```python
from build123d import *

# Parameters (mm, degrees)
SKETCH_1_W          = 18.3
SKETCH_1_H          = 42.85
SKETCH_1_R          = 1.55
EXTRUDE_1_DEPTH     = 7
SKETCH_2_W          = 5
SKETCH_2_H          = 14
EXTRUDE_4_DEPTH     = 8
SKETCH_5_W          = 5
SKETCH_5_H          = 3.15
EXTRUDE_5_DEPTH     = 35
EXTRUDE_7_DEPTH     = 35
EXTRUDE_8_DEPTH     = 5
CUT_EXTRUDE_1_REACH = 63.123
SKETCH_9_R          = 1.3
SKETCH_11_R         = 1.55
CUT_EXTRUDE_2_DEPTH = 32
SKETCH_12_W         = 6
SKETCH_12_H         = 6
CUT_EXTRUDE_3_DEPTH = 3.2
FILLET_1_R          = 5


with BuildPart() as part:
    # 草图1 → 凸台-拉伸1 (new body)
    with BuildSketch(Plane.XY):
        with Locations((9.15, -21.425)):
            Rectangle(SKETCH_1_W, SKETCH_1_H)
        with Locations((5.15, -5)):
            Circle(SKETCH_1_R, mode=Mode.SUBTRACT)
        with Locations((5.15, -37.96)):
            Circle(SKETCH_1_R, mode=Mode.SUBTRACT)
        with Locations(Location((13.15, -37.96, 0), (0, 0, 180))):
            Circle(SKETCH_1_R, mode=Mode.SUBTRACT)
        with Locations(Location((13.15, -5, 0), (0, 0, 180))):
            Circle(SKETCH_1_R, mode=Mode.SUBTRACT)
    extrude(amount=EXTRUDE_1_DEPTH)

    # 草图2 → 凸台-拉伸4 (add)
    with BuildSketch(Plane.XY.offset(7)):
        with Locations((15.8, -21.425)):
            Rectangle(SKETCH_2_W, SKETCH_2_H)
    extrude(amount=EXTRUDE_4_DEPTH)

    # 草图5 → 凸台-拉伸5 (add)
    with BuildSketch(Plane.XY.offset(7)):
        with Locations((15.8, -32.45)):
            Rectangle(SKETCH_5_W, SKETCH_5_H)
        with Locations((15.8, -10.4)):
            Rectangle(SKETCH_5_W, SKETCH_5_H)
    extrude(amount=EXTRUDE_5_DEPTH)

    # 草图7 → 凸台-拉伸7 (add)
    with BuildSketch(Plane.XY.offset(7)):
        Polygon((0, 0), (12.7, 0), (18.3, 0), (18.3, -8.825), (11.66, -8.825), (11.66, -34.025), (18.3, -34.025), (18.3, -42.85), (12.7, -42.85), (0, -42.85), align=None)
    extrude(amount=EXTRUDE_7_DEPTH)

    # 草图8 → 凸台-拉伸8 (add)
    with BuildSketch(Plane.XY.offset(7)):
        Polygon((13.3, -30.875), (13.3, -34.025), (11.66, -34.025), (11.66, -8.825), (13.3, -8.825), (13.3, -11.975), (18.3, -11.975), (18.3, -14.425), (13.3, -14.425), (13.3, -28.425), (18.3, -28.425), (18.3, -30.875), align=None)
    extrude(amount=EXTRUDE_8_DEPTH)

    # 草图9 → 切除-拉伸1 (cut, up to next)
    with BuildSketch(Plane(origin=(11.66, 0, 0), x_dir=(0, 0, -1), z_dir=(1, 0, 0)), mode=Mode.PRIVATE) as cut_extrude_1_sk1:
        with Locations(Location((-16.37, -13.195, 0), (0, 0, 90))):
            Circle(SKETCH_9_R)
    cut_extrude_1_tool1 = extrude(cut_extrude_1_sk1.sketch, amount=-CUT_EXTRUDE_1_REACH, mode=Mode.PRIVATE) & part.part
    # 草图9 → 切除-拉伸1 (cut, up to next)
    with BuildSketch(Plane(origin=(11.66, 0, 0), x_dir=(0, 0, -1), z_dir=(1, 0, 0)), mode=Mode.PRIVATE) as cut_extrude_1_sk2:
        with Locations((-16.37, -29.655)):
            Circle(SKETCH_9_R)
    cut_extrude_1_tool2 = extrude(cut_extrude_1_sk2.sketch, amount=-CUT_EXTRUDE_1_REACH, mode=Mode.PRIVATE) & part.part
    # 草图9 → 切除-拉伸1 (cut, up to next)
    with BuildSketch(Plane(origin=(11.66, 0, 0), x_dir=(0, 0, -1), z_dir=(1, 0, 0)), mode=Mode.PRIVATE) as cut_extrude_1_sk3:
        with Locations(Location((-32.63, -13.195, 0), (0, 0, 90))):
            Circle(SKETCH_9_R)
    cut_extrude_1_tool3 = extrude(cut_extrude_1_sk3.sketch, amount=-CUT_EXTRUDE_1_REACH, mode=Mode.PRIVATE) & part.part
    # 草图9 → 切除-拉伸1 (cut, up to next)
    with BuildSketch(Plane(origin=(11.66, 0, 0), x_dir=(0, 0, -1), z_dir=(1, 0, 0)), mode=Mode.PRIVATE) as cut_extrude_1_sk4:
        with Locations((-32.63, -29.655)):
            Circle(SKETCH_9_R)
    cut_extrude_1_tool4 = extrude(cut_extrude_1_sk4.sketch, amount=-CUT_EXTRUDE_1_REACH, mode=Mode.PRIVATE) & part.part
    add(cut_extrude_1_tool1.solids().sort_by_distance((11.66, -13.195, 16.37))[0], mode=Mode.SUBTRACT)
    add(cut_extrude_1_tool2.solids().sort_by_distance((11.66, -29.655, 16.37))[0], mode=Mode.SUBTRACT)
    add(cut_extrude_1_tool3.solids().sort_by_distance((11.66, -13.195, 32.63))[0], mode=Mode.SUBTRACT)
    add(cut_extrude_1_tool4.solids().sort_by_distance((11.66, -29.655, 32.63))[0], mode=Mode.SUBTRACT)

    # 草图11 → 切除-拉伸2 (cut)
    with BuildSketch(Plane(origin=(0, 0, 0), x_dir=(-1, 0, 0), z_dir=(0, 0, -1))):
        with Locations((-13.15, -5)):
            Circle(SKETCH_11_R)
        with Locations((-5.15, -5)):
            Circle(SKETCH_11_R)
        with Locations((-5.15, -37.96)):
            Circle(SKETCH_11_R)
        with Locations((-13.15, -37.96)):
            Circle(SKETCH_11_R)
    extrude(amount=-CUT_EXTRUDE_2_DEPTH, mode=Mode.SUBTRACT)

    # 草图12 → 切除-拉伸3 (cut)
    with BuildSketch(Plane.XY.offset(25)):
        with Locations((13.15, -5)):
            Rectangle(SKETCH_12_W, SKETCH_12_H)
        with Locations((5.15, -5)):
            Rectangle(SKETCH_12_W, SKETCH_12_H)
        with Locations((13.15, -37.96)):
            Rectangle(SKETCH_12_W, SKETCH_12_H)
        with Locations((5.15, -37.96)):
            Rectangle(SKETCH_12_W, SKETCH_12_H)
    extrude(amount=-CUT_EXTRUDE_3_DEPTH, mode=Mode.SUBTRACT)

    # 圆角1
    fillet_1_edges = [part.edges().sort_by_distance(p)[0] for p in [
        (9.15, -42.85, 42),
        (18.3, 0, 21),
        (18.3, -42.85, 21),
        (9.15, 0, 42),
    ]]
    fillet(fillet_1_edges, radius=FILLET_1_R)


solid = part.part
```
The model under review builds one solid part; all positions refer to its coordinate system, in mm. A direction names the side the tool comes from. Round coordinates to 2 decimals unless told otherwise and drop trailing zeros. Order: outer loops, then holes, each group sorted by start corner. A loop starts at its lowest first (then second) coordinate and runs counter-clockwise, first axis right, second up.
Item 1: Add section A-A, the plane z = 20.5. State the section outline as (x, y) points (3 decimals), and give its area (3 significant figures).
Working result:
outline: (0, -42.85) - (13.3, -42.85) arc R5 ccw to (18.3, -37.85) - (18.3, -30.875) - (13.3, -30.875) - (13.3, -34.025) - (11.66, -34.025) - (11.66, -8.825) - (13.3, -8.825) - (13.3, -11.975) - (18.3, -11.975) - (18.3, -5) arc R5 ccw to (13.3, 0) - (0, 0) - close; hole circle Ø3.1 at (5.15, -37.96); hole circle Ø3.1 at (5.15, -5); hole circle Ø3.1 at (13.15, -37.96); hole circle Ø3.1 at (13.15, -5)
area: 607 mm2
Item 2: Add section D-D, the plane x = 4.5. Count the separate pieces of the cut face and the enclosed holes in it, and give its area (3 significant figures).
Working result:
separate pieces: 1
enclosed holes: 4
area: 1,570 mm2
Item 3: Add section B-B, the plane z = 32.63. State the section outline as (x, y) points (3 decimals).
Working result:
outline: (0, -42.85) - (13.3, -42.85) arc R5 ccw to (18.3, -37.85) - (18.3, -30.875) - (13.3, -30.875) - (13.3, -34.025) - (11.66, -34.025) - (11.66, -30.955) - (0, -30.955) - close; (0, -28.355) - (11.66, -28.355) - (11.66, -14.495) - (0, -14.495) - close; (0, -11.895) - (11.66, -11.895) - (11.66, -8.825) - (13.3, -8.825) - (13.3, -11.975) - (18.3, -11.975) - (18.3, -5) arc R5 ccw to (13.3, 0) - (0, 0) - close
Item 4: Machinability: for faces 4 (the flat face through (5, -5, 32)), 5 (the flat face through (12, -34.025, 27)), 6 (the flat face through (16, -30.875, 27)), 7 (the flat face through (0, -22, 21)), 8 (the flat face through (11.8, -36.6, 25)), which of the approach directions +Z, -Z, +X, -X, +Y, -Y give a long, thin tool a straight path to every point of the face, cutting with its end or side? Answer none if there is none.
Working result:
face 4: -Z
face 5: +Z
face 6: +Z, +X
face 7: +Z, -Z, -X, +Y, -Y
face 8: none
Item 5: Add section C-C, the plane y = -21. State the section outline as (x, z) points, and give its area (3 significant figures).
Working result:
outline: (0, 0) - (18.3, 0) - (18.3, 15) - (13.3, 15) - (13.3, 12) - (11.66, 12) - (11.66, 42) - (0, 42) - close
area: 584 mm2
Item 6: Draft analysis for pull direction X (two halves, no side actions). For faces 1 (the cylindrical face through (16.87, -1.5, 20.71)), 2 (the flat face through (13, -38, 32)), 3 (the flat face through (16, -21, 15)), state which applies: released by +X, released by -X, zero draft, split by the parting line, or undercut.
Working result:
face 1: released by +X
face 2: undercut
face 3: zero draft
Item 7: For pin 1 (5.5 mm diameter, centred on x = 15.5, z = 25, fed in from +Y); pin 2 (8 mm diameter, centred on y = -19.5, z = 26, fed in from +X); pin 3 (2.5 mm diameter, centred on x = 15, z = 22.5, fed in from -Y); pin 4 (3 mm diameter, centred on x = 16, z = 14.5, fed in from -Y), all flat-tipped, find the tip position at first contact; note any pin that passes through.
Working result:
pin 1: stops at y = 0
pin 2: stops at x = 11.66
pin 3: stops at y = -42.83
pin 4: stops at y = -42.7
Item 8: To check wall thickness, follow probe 1 along Y at (x, z) = (5.25, 26.5); probe 2 along Z at (x, y) = (3.25, -29.5); probe 3 along Y at (x, z) = (13.15, 28) (3 decimals). State the ranges of each line that lie inside material, in increasing order.
Working result:
probe 1: y = -42.85 to -39.51, -36.41 to -6.55, -3.45 to 0
probe 2: z = 0 to 15.08, 17.66 to 31.34, 33.92 to 42
probe 3: y = -42.85 to -39.51, -36.41 to -34.025, -8.825 to -6.55, -3.45 to 0
